The listing builds one solid part. Answer for the finished solid, in the listing's coordinates (mm). Face numbers are marked on the shaded views. A direction names the side the tool comes from. Coordinates: 2 decimals unless noted, no trailing zeros. Write each loop counter-clockwise with the first axis right and the second up, starting at its lowest first coordinate (ties: lowest second). Pieces come first, ordered by that corner, then holes. Notation, with made-up numbers: M -16.5,0 L 28.5,0 A15 cw 28.5,13 Z; hole C 54,-5.5 d10. An arc over 180 degrees is marked long. Put each result on its own line as item: value. Start each with the question number.
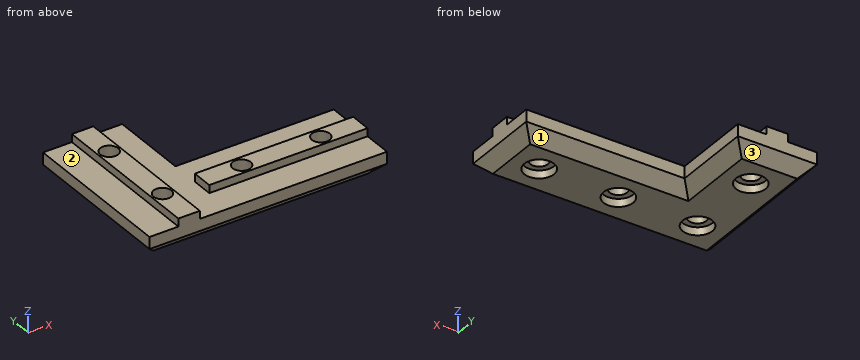
```python
from build123d import *

# Parameters (mm, degrees)
F1_DEPTH = 6
F3_DEPTH = 2
F4_R     = 2.25
F5_DEPTH = 8.001
F6_R     = 3.75
F7_DEPTH = 2
F8_SIZE  = 3


with BuildPart() as f1:
    # F0 (on Top) → F1 (new body)
    with BuildSketch(Plane.XY):
        Polygon((0, 40), (0, 0), (60, 0), (60, 20), (20, 20), (20, 40), align=None)
    extrude(amount=F1_DEPTH)

    # F2 (on face) → F3 (join)
    with BuildSketch(Plane.XY.offset(6)):
        Polygon((12.71, 40), (7.29, 40), (7.29, 0), (10, 0), (12.71, 0), align=None)
        Polygon((60, 7.29), (60, 12.71), (20, 12.71), (20, 10), (20, 7.29), align=None)
    extrude(amount=F3_DEPTH)

    # F4 (on face) → F5 (cut, through all)
    with BuildSketch(Plane(origin=(0, 0, 0), x_dir=(1, 0, 0), z_dir=(0, 0, -1))):
        with Locations((10, -10)):
            Circle(F4_R)
        with Locations((50, -10)):
            Circle(F4_R)
        with Locations((10, -30)):
            Circle(F4_R)
        with Locations((30, -10)):
            Circle(F4_R)
    extrude(amount=-F5_DEPTH, mode=Mode.SUBTRACT)

    # F6 (on face) → F7 (cut)
    with BuildSketch(Plane(origin=(0, 0, 0), x_dir=(1, 0, 0), z_dir=(0, 0, -1))):
        with Locations((10, -10)):
            Circle(F6_R)
        with Locations((30, -10)):
            Circle(F6_R)
        with Locations((50, -10)):
            Circle(F6_R)
        with Locations((10, -30)):
            Circle(F6_R)
    extrude(amount=-F7_DEPTH, mode=Mode.SUBTRACT)

    # F8
    f8_edges = [f1.edges().sort_by_distance(p)[0] for p in [
        (30, 0, 0),
        (0, 20, 0),
        (20, 30, 0),
        (40, 20, 0),
        (60, 10, 0),
        (10, 40, 0),
    ]]
    chamfer(f8_edges, length=F8_SIZE)


solid = f1.part
```
1) For the marked faces 1, 2 and 3, determine the directions among +Z, -Z, +X, -X, +Y, -Y from which every point of the face is accessible in a straight line to the end or side of a thin tool.
2) Straight lines are drawn through the part: probe 1 along Y at (x, z) = (10, 5.1); probe 2 along Y at (x, z) = (50, 4.7); probe 3 along X at (y, z) = (10, 0.75). For each, find the intervals that lie inside material, in ascending order.
3) Given pin 1 Ø1.5 at (x, z) = (40.5, 5) entering from +Y; pin 2 Ø6 at (x, y) = (10, 10) entering from -Z; pin 3 Ø0.6 at (y, z) = (27, 7.5) entering from -X; pin 4 Ø4 at (x, y) = (10, 30) entering from -Z, each flat-ended and moving along its own axis, determine where each tip first touches the part or whether it passes through.
4) A cutting plane is placed at A-A on z = 7.25. Write down the section's boundary in (x, y), then the cut area to 3 significant figures.
5) A cutting plane is placed at B-B on x = 50. Write down the section's boundary in (y, z).
6) A cutting plane is placed at D-D on x = 10. Write down the section's boundary in (y, z).
Answers follow:
1. face 1: -Z, +X, +Y
1. face 2: +Z, -X, +Y, -Y
1. face 3: -Z, +X, -X, +Y
2. probe 1: y = 0 to 7.75, 12.25 to 27.75, 32.25 to 40
2. probe 2: y = 0 to 7.75, 12.25 to 20
2. probe 3: x = 2.25 to 6.25, 13.75 to 26.25, 33.75 to 46.25, 53.75 to 57.75
3. pin 1: stops at y = 20
3. pin 2: stops at z = 2
3. pin 3: stops at x = 7.29
3. pin 4: passes through
4. outline: M 7.29,0 L 12.71,0 L 12.71,40 L 7.29,40 Z; M 20,7.29 L 60,7.29 L 60,12.71 L 20,12.71 Z; hole C 10,10 d4.5; hole C 10,30 d4.5; hole C 30,10 d4.5; hole C 50,10 d4.5
4. area: 370 mm²
5. outline: M 0,3 L 3,0 L 6.25,0 L 6.25,2 L 7.75,2 L 7.75,8 L 7.29,8 L 7.29,6 L 0,6 Z; M 12.25,2 L 13.75,2 L 13.75,0 L 17,0 L 20,3 L 20,6 L 12.71,6 L 12.71,8 L 12.25,8 Z
6. outline: M 0,3 L 3,0 L 6.25,0 L 6.25,2 L 7.75,2 L 7.75,8 L 0,8 Z; M 12.25,2 L 13.75,2 L 13.75,0 L 26.25,0 L 26.25,2 L 27.75,2 L 27.75,8 L 12.25,8 Z; M 32.25,2 L 33.75,2 L 33.75,0 L 37,0 L 40,3 L 40,8 L 32.25,8 Z
